For this review, use the dimensioned drawing (mm, ordinates from the lowest corner) and the shaded views. A direction names the side the tool comes from. Round coordinates to 2 decimals unless told otherwise and drop trailing zeros. Write each loop counter-clockwise with the first axis right and the second up, starting at its lowest first coordinate (ties: lowest second). Pieces come first, ordered by that corner, then holes. Notation, with made-up numbers: (-31.75, 84) - (21.25, 84) arc R23 ccw to (21.25, 97) - close; hole circle Ø9 at (-32.75, 30). An arc over 180 degrees is marked (long way). Write each question's results on one line, items separated by ' | '.
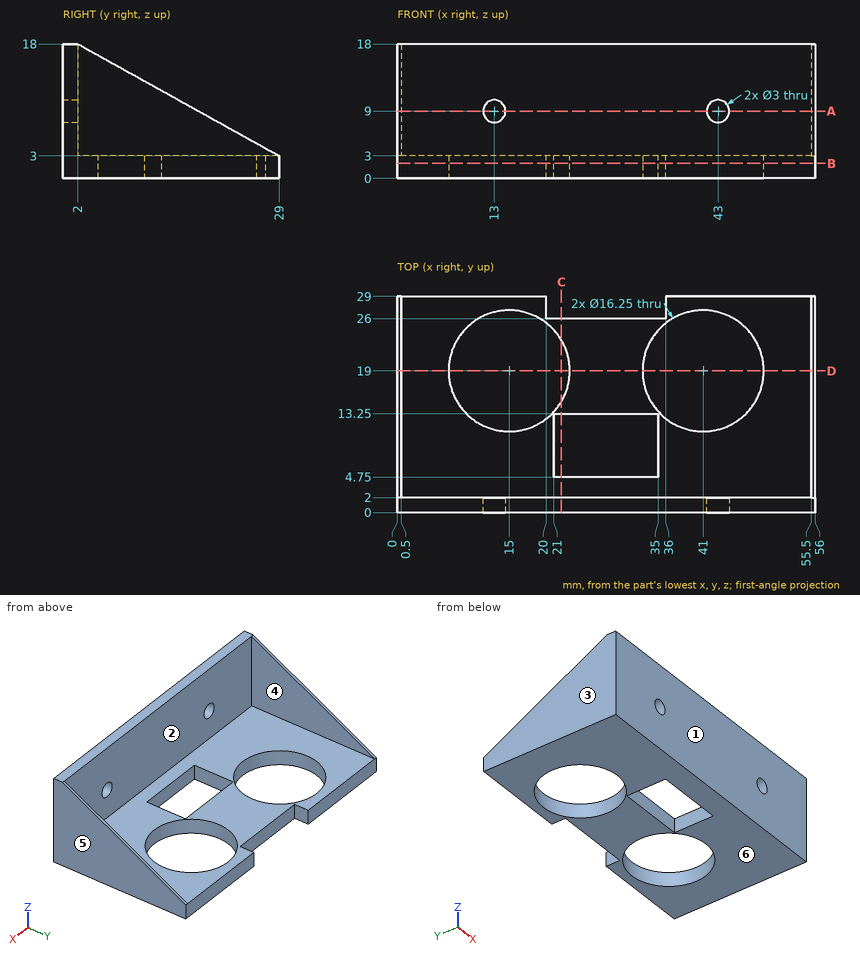
Q1. We need section C-C (x = 22). State the section outline as (y, z) points (3 decimals).
Evaluation:
outline: (0, 0) - (4.75, 0) - (4.75, 3) - (2, 3) - (2, 18) - (0, 18) - close; (13.25, 0) - (14.875, 0) - (14.875, 3) - (13.25, 3) - close; (23.125, 0) - (26, 0) - (26, 3) - (23.125, 3) - close
Q2. For probe 1 along Z at (x, y) = (13, 1.45); probe 2 along X at (y, z) = (7.75, 13.5); probe 3 along Y at (x, z) = (41, 1.3) (3 decimals), list the stretches that pass through material, from the lowest coordinate up.
Evaluation:
probe 1: z = 0 to 7.5, 10.5 to 18 | probe 2: x = 0 to 0.5, 55.5 to 56 | probe 3: y = 0 to 10.875, 27.125 to 29
Q3. We need section D-D (y = 19). State the section outline as (x, z) points (3 decimals), plus the area to 3 significant figures.
Evaluation:
outline: (0, 0) - (6.875, 0) - (6.875, 3) - (0.5, 3) - (0.5, 8.556) - (0, 8.556) - close; (23.125, 0) - (32.875, 0) - (32.875, 3) - (23.125, 3) - close; (49.125, 0) - (56, 0) - (56, 8.556) - (55.5, 8.556) - (55.5, 3) - (49.125, 3) - close | area: 76.1 mm^2
Q4. We need section A-A (z = 9). State the section outline as (x, y) points.
Evaluation:
outline: (0, 0) - (11.5, 0) - (11.5, 2) - (0.5, 2) - (0.5, 18.2) - (0, 18.2) - close; (14.5, 0) - (41.5, 0) - (41.5, 2) - (14.5, 2) - close; (44.5, 0) - (56, 0) - (56, 18.2) - (55.5, 18.2) - (55.5, 2) - (44.5, 2) - close
Q5. The part is to be moulded in two halves that separate along X. For the marked faces 3, 4, 5 and 6, say which applies: released by +X, released by -X, zero draft, split by the parting line, or undercut.
Evaluation:
face 3: released by -X | face 4: undercut | face 5: released by +X | face 6: zero draft
Q6. Insertion check: P1, Ø3, axis at y = 25, z = 7.5, coming from the -X side; P2, Ø2, axis at x = 33.5, z = 12.5, coming from the +Y side; P3, Ø2, axis at x = 7, y = 22, coming from the +Z side; P4, Ø3.5, axis at x = 25, z = 1.5, coming from the +Y side. Each pin has a flat end and moves straight along its axis. Give the tip position at first contact, or say it passes through.
Evaluation:
P1: passes through | P2: stops at y = 2 | P3: stops at z = 3 | P4: stops at y = 26
Q7. Tool access review of the marked faces 1 and 2: name each direction out of +Z, -Z, +X, -X, +Y, -Y from which nothing blocks a thin tool from reaching the whole face with its end or side.
Evaluation:
face 1: +Z, -Z, +X, -X, -Y | face 2: +Z, +Y
Q8. We need section B-B (z = 2). State the section outline as (x, y) points (3 decimals), plus the area to 3 significant figures.
Evaluation:
outline: (0, 0) - (56, 0) - (56, 29) - (36, 29) - (36, 26) - (20, 26) - (20, 29) - (0, 29) - close; hole circle Ø16.25 at (15, 19); hole (21, 4.75) - (35, 4.75) - (35, 13.25) - (21, 13.25) - close; hole circle Ø16.25 at (41, 19) | area: 1,040 mm^2
